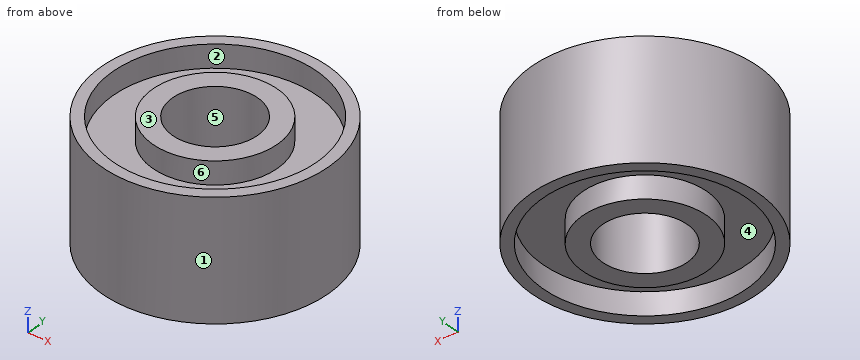
Autodesk Inventor part; units mm, degrees
ref_plane "Work Plane1" through (0, 0, 2.1) normal (0, 0, 1) x (1, 0, 0)
ref_plane "Work Plane2" through (0, 0, -2.1) normal (0, 0, -1) x (-1, 0, 0)
ref_plane "YZ Plane" through (0, 0, 0) normal (1, 0, 0) x (0, 1, 0)
sketch "Sketch1" plane through (0, 0, 0) normal (0, 0, 1) x (1, 0, 0)
  circle A0 centre (0, 0) radius 1.5
  circle A1 centre (0, 0) radius 2.2
  circle A2 centre (0, 0) radius 4
  dimension "d0" = 3
  dimension "d1" = 4.4
  dimension "d2" = 8
extrude "Extrusion1" add sketch "Sketch1" along normal mid plane 4.2 contours A1 | A2
ref_plane "Work Plane1" through (0, 0, 2.1) normal (0, 0, 1) x (1, 0, 0)
sketch "Sketch2" plane through (0, 0, 2.1) normal (0, 0, 1) x (1, 0, 0)
  circle A0 centre (0, 0) radius 2.2
  circle A1 centre (0, 0) radius 3.6
  dimension "d6" = 4.4
  dimension "d7" = 7.2
extrude "Extrusion2" cut sketch "Sketch2" against normal blind 0.8
ref_plane "Work Plane2" through (0, 0, -2.1) normal (0, 0, -1) x (-1, 0, 0)
sketch "Sketch3" plane through (0, 0, -2.1) normal (0, 0, -1) x (-1, 0, 0)
  circle A0 centre (0, 0) radius 3.6
  circle A1 centre (0, 0) radius 2.2
extrude "Extrusion3" cut sketch "Sketch3" against normal blind 0.8
properties part number "New_main_wheel"
Could you check a few things on this model? Use its own coordinates, in mm. Face numbers are marked on the shaded views. A direction names the side the tool comes from. Coordinates: 2 decimals unless noted, no trailing zeros. Order: outer loops, then holes, each group sorted by start corner. A loop starts at its lowest first (then second) coordinate and runs counter-clockwise, first axis right, second up. Notation, with made-up numbers: (-36.5, -37.5) -> (-22.5, -37.5) arc R21 cw to (-22.5, -25.5) -> close; hole circle Ø7 at (-19.5, 85.5). An arc over 180 degrees is marked (long way). One line per question, with ' | ' between items.
Q1. Thinking about a two-plate mould opening in X: for the marked faces 1, 2 and 3, which applies, pulls with the +X half, pulls with the -X half, needs draft (parallel to the pull), parting line crosses it, or undercut?
Return value:
face 1: parting line crosses it | face 2: undercut | face 3: needs draft
Q2. Imagine slicing it at C-C on z = 1.55. Please give me the cut outline in (x, y).
Return value:
outline: circle Ø8 at (0, 0); circle Ø4.4 at (0, 0); hole circle Ø7.2 at (0, 0); hole circle Ø3 at (0, 0)
Q3. On a 3-axis mill with a long thin cutter (end or side, diameter ignored), from which of +Z, -Z, +X, -X, +Y, -Y can I reach the whole of each face in a straight line? I mean the marked faces 4, 5 and 6. Say none if no direction works.
Return value:
face 4: -Z | face 5: +Z, -Z | face 6: +Z
Q4. I'm going to push flat-ended pins straight in: P1, Ø1, axis at x = -2, z = -1.5, coming from the -Y side; P2, Ø1, axis at x = -0.5, y = -3, coming from the +Z side; P3, Ø1, axis at y = 1, z = -1.5, coming from the +X side. Where does each tip first touch, or does it pass through?
Return value:
P1: y = -3.71 | P2: z = 1.3 | P3: x = 3.97
Q5. Imagine slicing it at A-A on x = 0. Please give me the cut outline in (y, z).
Return value:
outline: (-4, -2.1) -> (-3.6, -2.1) -> (-3.6, -1.3) -> (-2.2, -1.3) -> (-2.2, -2.1) -> (-1.5, -2.1) -> (-1.5, 2.1) -> (-2.2, 2.1) -> (-2.2, 1.3) -> (-3.6, 1.3) -> (-3.6, 2.1) -> (-4, 2.1) -> close; (1.5, -2.1) -> (2.2, -2.1) -> (2.2, -1.3) -> (3.6, -1.3) -> (3.6, -2.1) -> (4, -2.1) -> (4, 2.1) -> (3.6, 2.1) -> (3.6, 1.3) -> (2.2, 1.3) -> (2.2, 2.1) -> (1.5, 2.1) -> close
Q6. Imagine slicing it at D-D on z = -0.1. Please give me the cut outline in (x, y).
Return value:
outline: circle Ø8 at (0, 0); hole circle Ø3 at (0, 0)
Q7. If I drill on L1, parallel to Y at x = 0, z = 1.9; L2, parallel to Y at x = 0, z = -0.75; L3, parallel to Y at x = 0.5, z = -1.85, over which ranges is the centre line in solid material (lowest first)?
Return value:
L1: -4 to -3.6, -2.2 to -1.5, 1.5 to 2.2, 3.6 to 4 | L2: -4 to -1.5, 1.5 to 4 | L3: -3.97 to -3.57, -2.14 to -1.41, 1.41 to 2.14, 3.57 to 3.97
